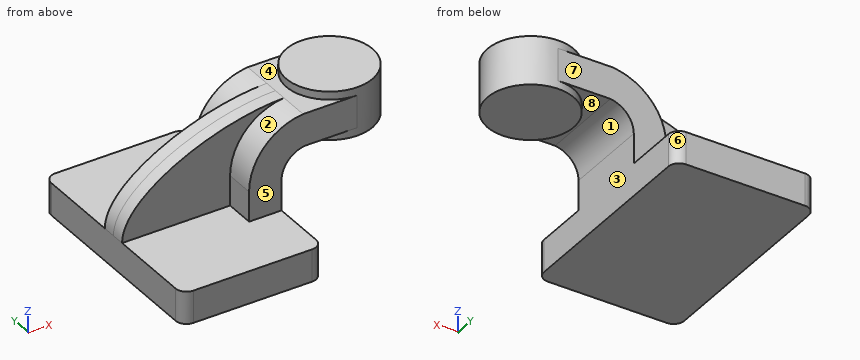
from build123d import *

# Parameters (mm, degrees)
F1_DEPTH = 63.5
F0_W     = 25.4
F0_H     = 19.05
F2_DEPTH = 25.4
F3_DEPTH = 7.9375
F5_R     = 6.35


with BuildPart() as f1:
    # F0 (on Front) → F1 (new body, symmetric)
    with BuildSketch(Plane.XZ):
        Polygon((22.225, 9.525), (-41.275, 9.525), (-41.275, -9.525), (41.275, -9.525), (41.275, 9.525), align=None)
    extrude(amount=F1_DEPTH, both=True)

    # F0 (on Front) → F2 (join, symmetric)
    with BuildSketch(Plane.XZ):
        with Locations((73.025, 52.4002)):
            Rectangle(F0_W, F0_H)
        with BuildLine():
            Line((22.225, 27.1454148694), (22.225, 9.525))
            Line((22.225, 9.525), (41.275, 9.525))
            Line((41.275, 9.525), (41.275, 27.1454148694))
            ThreePointArc((41.275, 27.1454148694), (45.1912214489, 37.5858765721), (55.0076917247, 42.8752))
            Line((55.0076917247, 42.8752), (60.325, 42.8752))
            Line((60.325, 42.8752), (60.325, 61.9252))
            Line((60.325, 61.9252), (53.9684640074, 61.9252))
            ThreePointArc((53.9684640074, 61.9252), (31.3539657162, 50.6894213303), (22.225, 27.1454148694))
        make_face()
    extrude(amount=F2_DEPTH, both=True)

    # F0 (on Front) → F3 (join, symmetric)
    with BuildSketch(Plane.XZ):
        with BuildLine():
            add(Edge.make_bspline(
                [(-41.275, 9.525), (-41.3264594972, 35.7253178954), (13.0891343579, 61.1484050751), (53.9684640074, 61.9252)],
                knots=[0, 0, 0, 0, 108.7064781702, 108.7064781702, 108.7064781702, 108.7064781702], degree=3))
            Line((-41.275, 9.525), (22.225, 9.525))
            Line((22.225, 9.525), (22.225, 27.1454148694))
            ThreePointArc((22.225, 27.1454148694), (31.3539657162, 50.6894213303), (53.9684640074, 61.9252))
        make_face()
    extrude(amount=F3_DEPTH, both=True)

    # F0 (on Front) → F4 (revolve)
    with BuildSketch(Plane.XZ):
        Polygon((85.725, 66.675), (85.725, 61.9252), (85.725, 42.8752), (85.725, 38.1), (111.125, 38.1), (111.125, 66.675), align=None)
    revolve(axis=Axis((85.725, 0, 52.3875), (0, 0, 1)))

    # F5
    f5_edges = [f1.edges().sort_by_distance(p)[0] for p in [
        (41.275, -63.5, 0),
        (-41.275, -63.5, 0),
        (41.275, 63.5, 0),
        (-41.275, 63.5, 0),
    ]]
    fillet(f5_edges, radius=F5_R)


solid = f1.part
The listing builds one solid part. Answer for the finished solid, in the listing's coordinates (mm). Face numbers are marked on the shaded views. A direction names the side the tool comes from. Round coordinates to 2 decimals unless told otherwise and drop trailing zeros. Write each loop counter-clockwise with the first axis right and the second up, starting at its lowest first coordinate (ties: lowest second). Pieces come first, ordered by that corner, then holes. Notation, with made-up numbers: M -19,78.25 L 25,78.25 A33 cw 25,110.25 Z; hole C 33,77.25 d3. An arc over 180 degrees is marked long. Write each question's results on one line, items separated by ' | '. Start each with the question number.
Item 1: A cutting plane is placed at D-D on y = 14. Write down the section's boundary in (x, z) (3 decimals).
Item 2: Straight lines are drawn through the part: L1, parallel to Z at x = 38, y = -51 (3 decimals); L2, parallel to Y at x = 11.5, z = 38; L3, parallel to Y at x = 40, z = 50. For each, find the intervals that lie inside material, in ascending order. Write a range as [from, to].
Item 3: Flat-ended cylindrical pins translate along their axes: pin 1 Ø18.5 at (y, z) = (0.5, 17.5) entering from +X (3 decimals); pin 2 Ø5 at (x, z) = (14, 16) entering from +Y; pin 3 Ø15.5 at (x, z) = (54, 29.5) entering from -Y; pin 4 Ø5 at (y, z) = (16.5, 21) entering from -X (3 decimals). Find the tip coordinate at first contact, or state that the pin passes through.
Item 4: A cutting plane is placed at A-A on z = -0.5. Write down the section's boundary in (x, y) (3 decimals).
Item 5: For a pull along X with two mould halves and no side action, classify the marked faces 6, 7 and 8 as pulls with the +X half, pulls with the -X half, needs draft (parallel to the pull), parting line crosses it, or undercut.
Item 6: A cutting plane is placed at C-C on x = 57. Write down the section's boundary in (y, z), and give its area (3 significant figures).
Item 7: A cutting plane is placed at B-B on y = -19. Write down the section's boundary in (x, z) (3 decimals), and give its area (3 significant figures).
Item 8: For the marked faces 1, 2, 3, 4 and 5, determine the directions among +Z, -Z, +X, -X, +Y, -Y from which every point of the face is accessible in a straight line to the end or side of a thin tool.
Check sheet entries:
1) outline: M -41.275,-9.525 L 41.275,-9.525 L 41.275,27.145 A15.875 cw 55.008,42.875 L 64.532,42.875 L 64.532,38.1 L 106.918,38.1 L 106.918,66.675 L 64.532,66.675 L 64.532,61.925 L 53.968,61.925 A34.925 ccw 22.225,27.145 L 22.225,9.525 L -41.275,9.525 Z
2) L1: [-9.525, 9.525] | L2: [-7.94, 7.94] | L3: [-25.4, 25.4]
3) pin 1: x = 41.275 | pin 2: y = 7.94 | pin 3: through | pin 4: x = 22.225
4) outline: M -41.275,-57.15 A6.35 ccw -34.925,-63.5 L 34.925,-63.5 A6.35 ccw 41.275,-57.15 L 41.275,57.15 A6.35 ccw 34.925,63.5 L -34.925,63.5 A6.35 ccw -41.275,57.15 Z
5) face 6: pulls with the +X half | face 7: needs draft | face 8: undercut
6) outline: M -25.4,42.88 L 25.4,42.88 L 25.4,61.93 L -25.4,61.93 Z | area: 968 mm²
7) outline: M -41.275,-9.525 L 41.275,-9.525 L 41.275,27.145 A15.875 cw 55.008,42.875 L 68.868,42.875 L 68.868,38.1 L 102.582,38.1 L 102.582,66.675 L 68.868,66.675 L 68.868,61.925 L 53.968,61.925 A34.925 ccw 22.225,27.145 L 22.225,9.525 L -41.275,9.525 Z | area: 3,850 mm²
8) face 1: -Z, +Y, -Y | face 2: +Z, -X, -Y | face 3: -Z, +X, +Y, -Y | face 4: +Z, -X | face 5: +Z, +X, -X, -Y
